The listing builds one solid part. Answer for the finished solid, in the listing's coordinates (mm). Face numbers are marked on the shaded views. A direction names the side the tool comes from. Give positions to 0.01 mm unless a question says otherwise; leave off trailing zeros. Loops run counter-clockwise (first coordinate to the right, second up) from the corner with the lowest first, then second, coordinate; pieces in that order, holes last. Notation, with made-up numbers: (79, 52) - (132, 52) arc R15 cw to (132, 60) - close; hole circle Ø5 at (58.5, -37). An arc over 180 degrees is marked (long way). Answer in a Markdown table with one row per item. Add a question column.
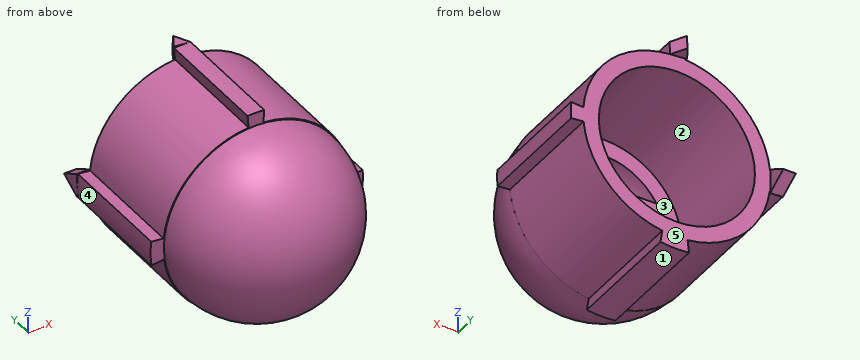
```python
from build123d import *

# Parameters (mm, degrees)
SKETCH1_R           = 12.5
BOSS_EXTRUDE1_DEPTH = 19
REVOLVE_THIN8_ANGLE = 180
BOSS_EXTRUDE4_DEPTH = 2
BOSS_EXTRUDE5_DEPTH = 2


# Read off the part's stored shape, not the designer's step: Revolve-Thin8
with BuildPart() as part:
    # Sketch1 → Boss-Extrude1 (new body)
    with BuildSketch(Plane(origin=(0, 0, 0), x_dir=(1, 0, 0), z_dir=(0, 1, 0))):
        with BuildLine():
            Line((-16.857907097, 2.193391967), (-14.874623909, 1.935345853))
            ThreePointArc((-14.874623909, 1.935345853), (-10.527218249, 10.68539545), (-1.713310211, 14.901831032))
            Line((-1.713310211, 14.901831032), (-1.941751573, 16.888741837))
            ThreePointArc((-1.941751573, 16.888741837), (0.351548962, 16.996364709), (2.638437912, 16.794006234))
            Line((2.638437912, 16.794006234), (2.328033452, 14.818240795))
            ThreePointArc((2.328033452, 14.818240795), (10.955949894, 10.245348306), (14.940866835, 1.330600703))
            Line((14.940866835, 1.330600703), (16.932982413, 1.50801413))
            ThreePointArc((16.932982413, 1.50801413), (16.999139456, 0.171049014), (16.959898748, -1.166976638))
            Line((16.959898748, -1.166976638), (14.964616542, -1.029685269))
            ThreePointArc((14.964616542, -1.029685269), (10.617208635, -10.595984183), (1.059628295, -14.962526119))
            Line((1.059628295, -14.962526119), (1.200912068, -16.957529602))
            ThreePointArc((1.200912068, -16.957529602), (-0.131031268, -16.999495016), (-1.462169449, -16.937002701))
            Line((-1.462169449, -16.937002701), (-1.290149514, -14.944414148))
            ThreePointArc((-1.290149514, -14.944414148), (-10.511046509, -10.701303719), (-14.91886862, -1.557998423))
            Line((-14.91886862, -1.557998423), (-16.908051103, -1.765731546))
            ThreePointArc((-16.908051103, -1.765731546), (-16.998636652, 0.215295063), (-16.857907097, 2.193391967))
        make_face()
        with Locations(Location((0, 0, 0), (0, 0, 270))):
            Circle(SKETCH1_R, mode=Mode.SUBTRACT)
    extrude(amount=BOSS_EXTRUDE1_DEPTH)

    # Revolve-Thin8 outline → Revolve-Thin8 (revolve)
    with BuildSketch(Plane.ZX):
        with BuildLine():
            ThreePointArc((0, -14.874623909), (14.874623909, 0), (0, 14.874623909))
            Line((0, 14.874623909), (0, -14.874623909))
        make_face()
        with BuildLine():
            Line((5, -8.515174534), (5, 8.515174534))
            ThreePointArc((5, 8.515174534), (9.874623909, 0), (5, -8.515174534))
        make_face(mode=Mode.SUBTRACT)
    revolve(axis=Axis((0, 0, 0), (1, 0, 0)), revolution_arc=REVOLVE_THIN8_ANGLE)

    # Sketch6 → Boss-Extrude4 (add)
    with BuildSketch(Plane(origin=(1.200912068, 9.5, 16.957529602), x_dir=(0.9975017412997444, 0, -0.0706418863279974), z_dir=(0.0706418863279974, 0, 0.9975017412997444))):
        Polygon((0, 9.5), (-1.345294106, 11.830117743), (-2.690588212, 9.5), align=None)
    extrude(amount=-BOSS_EXTRUDE4_DEPTH)

    # Sketch7 → Boss-Extrude5 (add)
    with BuildSketch(Plane(origin=(-16.998636652, 0, -0.215295063), x_dir=(-0.012664415486466005, 0, 0.9999198030744196), z_dir=(-0.9999198030744197, 0, -0.012664415486466006))):
        Polygon((-1.921412098, 18.937041844), (2.005099018, 18.937041844), (0.04184346, 22.337500219), align=None)
    extrude(amount=-BOSS_EXTRUDE5_DEPTH)


solid = part.part
```
(1) A cutting plane is placed at C-C on z = -7. Determine the outline of the cut face in (x, y).
(2) A cutting plane is placed at D-D on z = -3.5. Determine the outline of the cut face in (x, y).
(3) A cutting plane is placed at A-A on y = 11.5. Determine the outline of the cut face in (x, z).
(4) Find the intervals of material crossed by line 1 along Z through (x, y) = (0, 8); line 2 along Z through (x, y) = (-4.5, -2), in increasing order. Write a range as [from, to].
(5) A tool of negligible diameter and unlimited length cuts with its end or side. For the marked faces 1 and 2, from which of +Z, -Z, +X, -X, +Y, -Y can it reach the whole face along a straight path? Write none if from no direction.
(6) A cutting plane is placed at B-B on z = 4. Determine the outline of the cut face in (x, y).
(7) Given pin 1 Ø6 at (x, z) = (11.5, 7) entering from +Y; pin 2 Ø2 at (y, z) = (18.5, 7) entering from -X; pin 3 Ø12 at (y, z) = (-11, -5.5) entering from +X, each flat-ended and moving along its own axis, determine where each tip first touches the part or whether it passes through.
(8) The mould has two halves that part along Z. Classify the marked faces 3, 4 and 5: pulls with the +Z half, pulls with the -Z half, needs draft (parallel to the pull), parting line crosses it, or undercut.
Evaluation:
| question | item | result |
|---|---|---|
| 1 | outline | (-13.27, 0) - (-13.12, 0) arc R13.12 ccw to (13.12, 0) - (13.27, 0) - (13.27, 19) - (10.36, 19) - (10.36, 0) - (6.96, 0) arc R6.96 cw to (-6.96, 0) - (-10.36, 0) - (-10.36, 19) - (-13.27, 19) - close |
| 2 | outline | (-14.59, 0) - (-14.46, 0) arc R14.46 ccw to (14.46, 0) - (14.59, 0) - (14.59, 19) - (12, 19) - (12, 0) - (-12, 0) - (-12, 19) - (-14.59, 19) - close; hole (-8.52, -3.57) arc R9.23 ccw to (8.52, -3.57) - close |
| 3 | outline | (-16.91, 1.77) arc R17 ccw to (-16.86, -2.19) - (-14.87, -1.94) arc R15 ccw to (-1.71, -14.9) - (-1.94, -16.89) arc R17 ccw to (2.64, -16.79) - (2.33, -14.82) arc R15 ccw to (14.94, -1.33) - (16.93, -1.51) arc R17 ccw to (16.96, 1.17) - (14.96, 1.03) arc R15 ccw to (1.06, 14.96) - (1.2, 16.96) arc R17 ccw to (-1.46, 16.94) - (-1.29, 14.94) arc R15 ccw to (-14.92, 1.56) - close; hole circle Ø25 at (0, 0) |
| 4 | line 1 | z = [-17, -12.5], [12.5, 17] |
| 4 | line 2 | z = [-14.04, -8.56], [-4.58, 4.58], [8.56, 14.04] |
| 5 | face 1 | -Z, +Y, -Y |
| 5 | face 2 | +Y |
| 6 | outline | (-14.46, 0) - (-14.33, 0) arc R14.33 ccw to (14.33, 0) - (14.46, 0) - (14.46, 19) - (11.84, 19) - (11.84, 0) - (-11.84, 0) - (-11.84, 19) - (-14.46, 19) - close; hole (-8.52, -3) arc R9.03 ccw to (8.52, -3) - close |
| 7 | pin 1 | stops at y = 19 |
| 7 | pin 2 | stops at x = -13.75 |
| 7 | pin 3 | stops at x = 13.48 |
| 8 | face 3 | undercut |
| 8 | face 4 | parting line crosses it |
| 8 | face 5 | needs draft |
